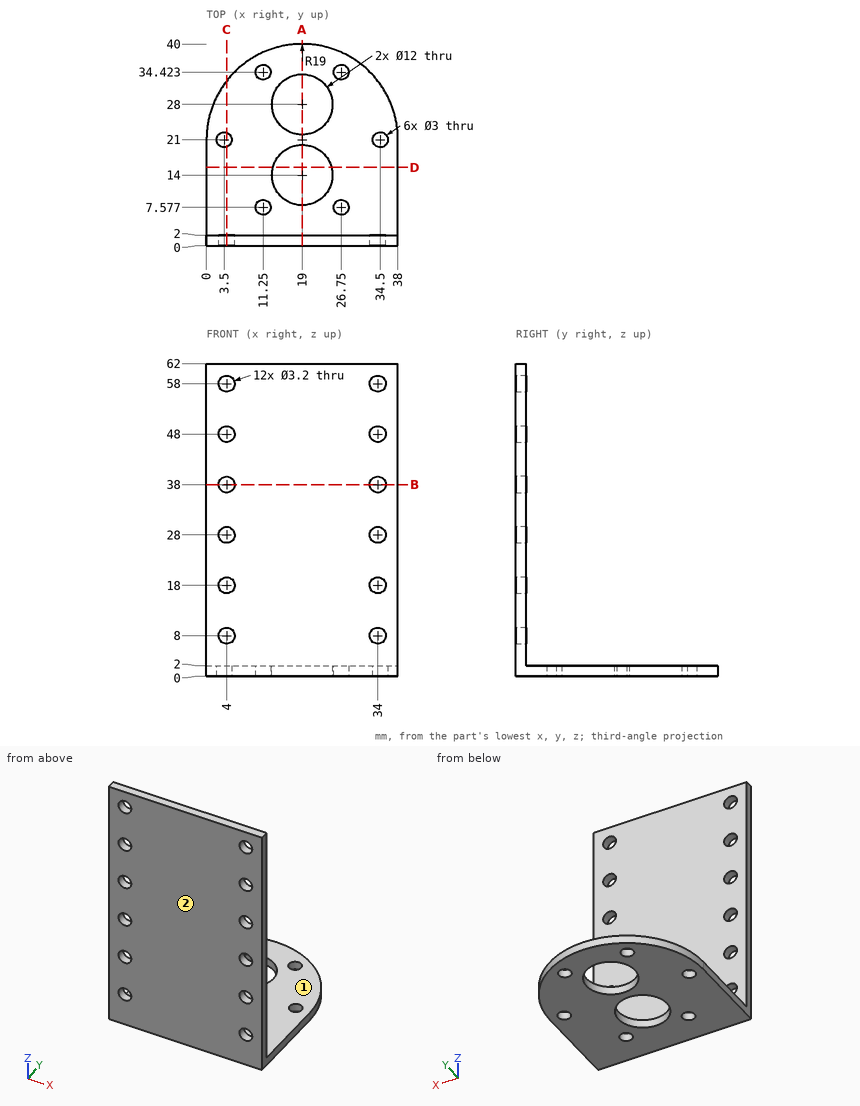
Job drawing, mm, ordinate dimensions from the low corner. One solid piece. A direction names the side the tool comes from. Coordinates: 2 decimals unless noted, no trailing zeros. Loops run counter-clockwise (first coordinate to the right, second up) from the corner with the lowest first, then second, coordinate; pieces in that order, holes last. Notation, with made-up numbers: (47.25, -5) - (96.25, -5) arc R19 cw to (96.25, 7) - close; hole circle Ø8 at (-27, 43.5). An arc over 180 degrees is marked (long way). Answer as a JSON object with one key per item and string values. Group by question number.
(1) Flat gauge pins, fed straight in: pin 1 (6 mm diameter, centred on x = 27, z = 48.5, fed in from +Y); pin 2 (2.5 mm diameter, centred on x = 34.5, y = 21, fed in from -Z); pin 3 (12 mm diameter, centred on x = 18.5, y = 22, fed in from +Z). Where does each tip first touch, or does it go through?
(2) Tool access for the marked faces 1 and 2: list every direction of +Z, -Z, +X, -X, +Y, -Y with a clear straight run to the whole face (end or side of a thin tool).
(3) Cut at A-A (x = 19). Give the cut face in (y, z), then the cut area to 3 significant figures.
(4) Cut at B-B (z = 38). Give the cut face in (x, y).
(5) Cut at C-C (x = 4). State how many separate pieces and enclosed holes the cut face has, then the cut area to 3 significant figures.
(6) Probe line 1 along X through (y, z) = (1, 8); line 2 along Y through (x, z) = (26.75, 1.4); line 3 along Y through (x, z) = (7, 13.5). List the from-to ranges inside material, lowest first.
(7) Cut at D-D (y = 15.5). Give the cut face in (x, z).
Geometry says:
{
 "1": {"pin 1": "stops at y = 2", "pin 2": "passes through", "pin 3": "stops at z = 2"},
 "2": {"face 1": "+Z, +X, -X, +Y", "face 2": "+Z, -Z, +X, -X, -Y"},
 "3": {"outline": "(0, 0) - (8, 0) - (8, 2) - (2, 2) - (2, 62) - (0, 62) - close; (20, 0) - (22, 0) - (22, 2) - (20, 2) - close; (34, 0) - (40, 0) - (40, 2) - (34, 2) - close", "area": "152 mm^2"},
 "4": {"outline": "(0, 0) - (2.4, 0) - (2.4, 2) - (0, 2) - close; (5.6, 0) - (32.4, 0) - (32.4, 2) - (5.6, 2) - close; (35.6, 0) - (38, 0) - (38, 2) - (35.6, 2) - close"},
 "5": {"separate pieces": "8", "enclosed holes": "0", "area": "141 mm^2"},
 "6": {"line 1": "x = 0 to 2.4, 5.6 to 32.4, 35.6 to 38", "line 2": "y = 0 to 6.08, 9.08 to 32.92, 35.92 to 38.35", "line 3": "y = 0 to 2"},
 "7": {"outline": "(0, 0) - (13.19, 0) - (13.19, 2) - (0, 2) - close; (24.81, 0) - (38, 0) - (38, 2) - (24.81, 2) - close"}
}
